Job drawing, mm, ordinate dimensions from the low corner. One solid piece. A direction names the side the tool comes from. Coordinates: 2 decimals unless noted, no trailing zeros. Loops run counter-clockwise (first coordinate to the right, second up) from the corner with the lowest first, then second, coordinate; pieces in that order, holes last. Notation, with made-up numbers: (67, -17.5) -> (80, -17.5) arc R8 cw to (80, -3.5) -> close; hole circle Ø6 at (-25, 3.25). An arc over 180 degrees is marked (long way). Use one line per item in the form item = value. Start each with the question number.
(1) Band-saw the part on A-A on y = 6.75. Give the cut face in (x, z) (1 decimal).
(2) Mould opens along X. For the marked faces 4, 5, 6 and 7 say: +X half, -X half, draft (parallel to the pull), parting line (faces both ways), or undercut.
(3) 3-axis set-ups, long thin cutter, end or side, ignore diameter. For the marked faces 1, 2 and 3: which of +Z, -Z, +X, -X, +Y, -Y reach the whole face in a straight line?
(4) Band-saw the part on C-C on z = 7.75. Give the cut face in (x, y) (1 decimal).
(5) Drill centre lines: L1, parallel to Z at x = 57, y = 8.5; L2, parallel to Z at x = 71, y = 13; L3, parallel to X at y = 9.25, z = 13.25 (1 decimal). Where is each one in solid material? Low to high. Write a range as [from, to].
(6) Pin check, flat tips, straight feed: P1, Ø7.5, axis at y = 10, z = 3.5, coming from the +X side; P2, Ø0.8, axis at y = 8.5, z = 21, coming from the -X side (1 decimal); P3, Ø8, axis at x = 68.5, y = 3.5, coming from the +Z side. Stop position of each tip, or through.
(7) Band-saw the part on B-B on x = 54. Give the cut face in (y, z) (1 decimal).
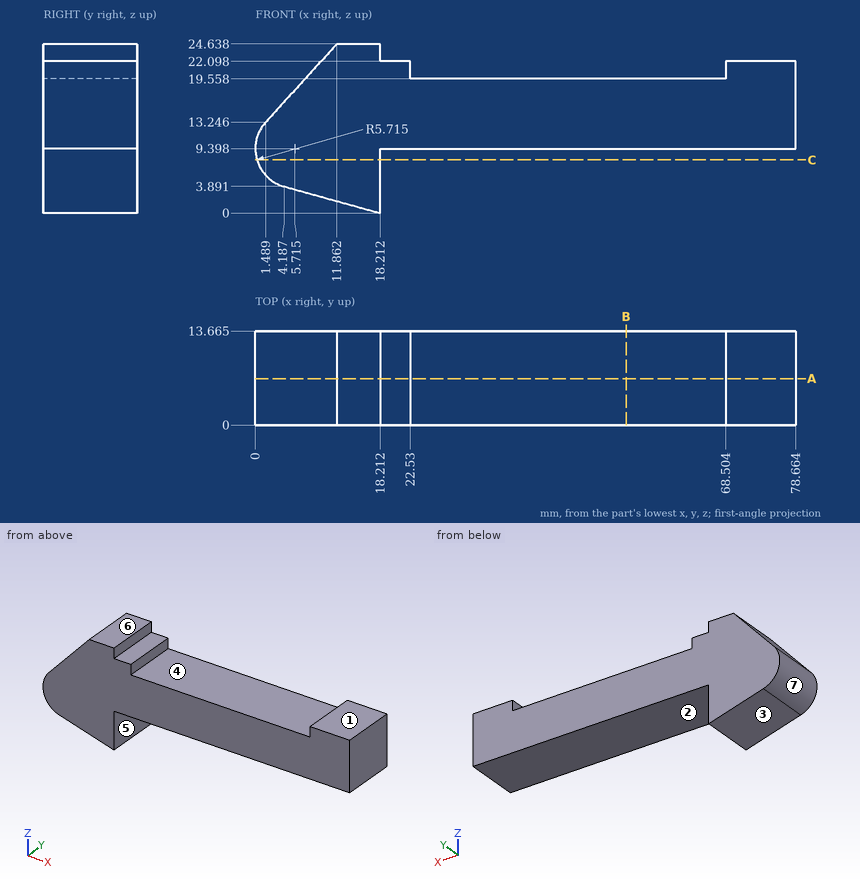
A:
q1.outline = (1.5, 13.2) arc R5.7 ccw to (4.2, 3.9) -> (18.2, 0) -> (18.2, 9.4) -> (78.7, 9.4) -> (78.7, 22.1) -> (68.5, 22.1) -> (68.5, 19.6) -> (22.5, 19.6) -> (22.5, 22.1) -> (18.2, 22.1) -> (18.2, 24.6) -> (11.9, 24.6) -> close
q2.face_4 = undercut
q2.face_5 = +X half
q2.face_6 = draft
q2.face_7 = -X half
q3.face_1 = +Z, +X, +Y, -Y
q3.face_2 = -Z, +X, +Y, -Y
q3.face_3 = -Z, -X, +Y, -Y
q4.outline = (0.2, 0) -> (18.2, 0) -> (18.2, 13.7) -> (0.2, 13.7) -> close
q5.L1 = [9.4, 19.56]
q5.L2 = [9.4, 22.1]
q5.L3 = [1.5, 78.7]
q6.P1 = 18.21
q6.P2 = 8.2
q6.P3 = 22.1
q7.outline = (0, 9.4) -> (13.7, 9.4) -> (13.7, 19.6) -> (0, 19.6) -> close
